Autodesk Inventor part; units mm, degrees
ref_plane "YZ Plane" through (0, 0, 0) normal (1, 0, 0) x (0, 1, 0)
ref_plane "XZ Plane" through (0, 0, 0) normal (0, 1, 0) x (-1, 0, 0)
ref_plane "XY Plane" through (0, 0, 0) normal (0, 0, 1) x (1, 0, 0)
sketch "Sketch1" plane through (0, 0, 0) normal (0, 1, 0) x (-1, 0, 0)
  line L0 (0, 3.1639) -> (2.74, 1.5819)
  line L1 (2.74, 1.5819) -> (2.74, -1.5819)
  line L2 (2.74, -1.5819) -> (0, -3.1639)
  line L3 (0, -3.1639) -> (-2.74, -1.5819)
  line L4 (-2.74, -1.5819) -> (-2.74, 1.5819)
  line L5 (-2.74, 1.5819) -> (0, 3.1639)
  point P0 (0, 0)
  point P1 (0, 0)
  dimension "d0" = 5.48
extrude "Extrusion1" add sketch "Sketch1" along normal blind 6.2
sketch "Sketch2" plane through (0, 6.2, 0) normal (0, 1, 0) x (1, 0, 0)
  circle A0 centre (0, 0) radius 1.5
  dimension "d3" = 3
extrude "Extrusion2" add sketch "Sketch2" along normal blind 6
thread "Thread1"
chamfer "Chamfer1" distance 0.3 angle 45 1 edges at (-1.5, 12.2, 0)
sketch "Sketch3" plane through (0, 0, 0) normal (0, -1, 0) x (1, 0, 0)
  circle A0 centre (0, 0) radius 1.5
  dimension "d11" = 3
extrude "Extrusion3" cut sketch "Sketch3" against normal blind 4.6
thread "Thread2"
chamfer "Chamfer2" distance 0.3 angle 45 1 edges at (-1.5, 0, 0)
properties part number "20mm_support"
Work out the finished part from the listing and answer in its coordinate system (mm). A direction names the side the tool comes from. Round coordinates to 2 decimals unless told otherwise and drop trailing zeros. Write each loop counter-clockwise with the first axis right and the second up, starting at its lowest first coordinate (ties: lowest second). Pieces come first, ordered by that corner, then holes. Notation, with made-up numbers: (61.25, 9.5) - (67.25, 9.5) arc R28 cw to (67.25, 41.5) - close; hole circle Ø5 at (65.5, 72). An arc over 180 degrees is marked (long way). Return JSON: item names as keys, results as strings. Group by question number.
Q1. The mould has two halves that part along Z. Classify faces 1 (the cylindrical face through (-1.5, 9.01, 0.07)), 2 (the flat face through (0, 4.6, 0)), 3 (the flat face through (0, 12.2, 0)), 4 (the cylindrical face through (-1.5, 2.42, 0.07)): released by +Z, released by -Z, zero draft, split by the parting line, or undercut.
Q2. The part is cut by section C-C on y = 11.25. Write down the section's boundary in (x, z), then the cut area to 3 significant figures.
Q3. The part is cut by section D-D on z = 2.75. Write down the section's boundary in (x, y).
Q4. For faces 5 (the flat face through (1.351, 3.057, -2.384)), 6 (the flat face through (1.3, 6.2, -1.4)), determine the directions among +Z, -Z, +X, -X, +Y, -Y from which every point of the face is accessible in a straight line to the end or side of a thin tool.
Q5. The part is cut by section B-B on z = 0. Write down the section's boundary in (x, y), then the cut area to 3 significant figures.
Q6. Find the intervals of material crossed by L1, parallel to Y at x = -0.6, z = -2; L2, parallel to X at y = 4, z = -0.25; L3, parallel to Z at x = 0.05, y = 9, in increasing order.
Q7. Each of these flat-tipped pins is pushed along its axis until it touches: pin 1 Ø2.5 at (x, z) = (-1, -1) entering from +Y; pin 2 Ø1.5 at (x, z) = (-0.5, 0.5) entering from -Y; pin 3 Ø2 at (x, y) = (0, 10.5) entering from +Z. Where does it stop, or does it pass through?
Q8. The part is cut by section A-A on y = 3.5. Write down the section's boundary in (x, z), then the cut area to 3 significant figures.
Solved:
{
 "1": {"face 1": "split by the parting line", "face 2": "undercut", "face 3": "zero draft", "face 4": "undercut"},
 "2": {"outline": "circle Ø3 at (0, 0)", "area": "7.07 mm²"},
 "3": {"outline": "(-0.72, 0) - (0.72, 0) - (0.72, 6.2) - (-0.72, 6.2) - close"},
 "4": {"face 5": "-Z, +X, +Y, -Y", "face 6": "+Y"},
 "5": {"outline": "(-2.74, 0) - (-1.8, 0) - (-1.5, 0.3) - (-1.5, 4.6) - (1.5, 4.6) - (1.5, 0.3) - (1.8, 0) - (2.74, 0) - (2.74, 6.2) - (1.5, 6.2) - (1.5, 11.9) - (1.2, 12.2) - (-1.2, 12.2) - (-1.5, 11.9) - (-1.5, 6.2) - (-2.74, 6.2) - close", "area": "38.0 mm²"},
 "6": {"L1": "0 to 6.2", "L2": "-2.74 to -1.48, 1.48 to 2.74", "L3": "-1.5 to 1.5"},
 "7": {"pin 1": "y = 12.2", "pin 2": "y = 4.6", "pin 3": "z = 1.5"},
 "8": {"outline": "(-2.74, -1.58) - (0, -3.16) - (2.74, -1.58) - (2.74, 1.58) - (0, 3.16) - (-2.74, 1.58) - close; hole circle Ø3 at (0, 0)", "area": "18.9 mm²"}
}
